from build123d import *

# Parameters (mm, degrees)
SKETCH1_W           = 51
SKETCH1_H           = 45
BOSS_EXTRUDE1_DEPTH = 5
SKETCH2_W           = 30
SKETCH2_H           = 30
BOSS_EXTRUDE2_DEPTH = 30
SKETCH3_W           = 20.5
SKETCH3_H           = 20.5
CUT_EXTRUDE1_DEPTH  = 38.5
SKETCH4_R           = 2.75
CUT_EXTRUDE2_DEPTH  = 36


with BuildPart() as part:
    # Sketch1 → Boss-Extrude1 (new body)
    with BuildSketch(Plane.XY):
        with Locations((0, -37.5)):
            Rectangle(SKETCH1_W, SKETCH1_H)
    extrude(amount=BOSS_EXTRUDE1_DEPTH)

    # Sketch2 → Boss-Extrude2 (add)
    with BuildSketch(Plane.XY.offset(5)):
        with Locations((0, -37.5)):
            Rectangle(SKETCH2_W, SKETCH2_H)
    extrude(amount=BOSS_EXTRUDE2_DEPTH)

    # Sketch3 → Cut-Extrude1 (cut, through all)
    with BuildSketch(Plane.XZ.offset(52.5)):
        with Locations((0, 20)):
            Rectangle(SKETCH3_W, SKETCH3_H)
    extrude(amount=-CUT_EXTRUDE1_DEPTH, mode=Mode.SUBTRACT)

    # Sketch4 → Cut-Extrude2 (cut, through all)
    with BuildSketch(Plane(origin=(0, 0, 0), x_dir=(-1, 0, 0), z_dir=(0, 0, -1))):
        with Locations((20, -37.5)):
            Circle(SKETCH4_R)
        with Locations((-20, -37.5)):
            Circle(SKETCH4_R)
    extrude(amount=-CUT_EXTRUDE2_DEPTH, mode=Mode.SUBTRACT)


solid = part.part
Model file for the job. Use its own axes, mm. A direction names the side the tool comes from. Give positions to 0.01 mm unless a question says otherwise; leave off trailing zeros. Loops run counter-clockwise (first coordinate to the right, second up) from the corner with the lowest first, then second, coordinate; pieces in that order, holes last. Notation, with made-up numbers: (-13, 80.5) -> (-4, 80.5) arc R7 ccw to (-4, 88.5) -> close; hole circle Ø2 at (18, 73.5). An arc over 180 degrees is marked (long way). Use a Markdown table: item, result. Add a question column.
(1) Wall check: line 1 along Z through (x, y) = (-8, -51); line 2 along X through (y, z) = (-39, 22.5); line 3 along Y through (x, z) = (20, 2). Give the ranges that are in metal, low to high.
(2) Slice it at D-D on y = -33. List the corners of the cut face in (x, z), and give its area (3 significant figures).
(3) Drop flat-ended pins along their axis: pin 1 Ø4 at (y, z) = (-47, 28.5) entering from -X; pin 2 Ø12 at (y, z) = (-42.5, 25.5) entering from +X; pin 3 Ø3 at (x, z) = (-11, 30) entering from +Y. Give the stop position or say it passes through.
(4) Mould opens along X. For faces 1 (the flat face through (0, -22, 5)), 2 (the flat face through (10.25, -38, 20)), 3 (the flat face through (25.5, -38, 2)) say: +X half, -X half, draft (parallel to the pull), parting line (faces both ways), or undercut.
(5) Slice it at B-B on x = -20. List the corners of the cut face in (y, z), and give its area (4 significant figures).
(6) Slice it at C-C on z = 22.5. List the corners of the cut face in (x, y), and give its area (3 significant figures).
(7) Tool access for faces 4 (the flat face through (15, -38, 20)), 5 (the flat face through (-15, -38, 20)), 6 (the flat face through (-10.25, -38, 20)): list every direction of +Z, -Z, +X, -X, +Y, -Y with a clear straight run to the whole face (end or side of a thin tool).
(8) Slice it at A-A on y = -37.5. List the corners of the cut face in (x, z), and give its area (3 significant figures).
Filled sheet:
| question | item | result |
|---|---|---|
| 1 | line 1 | 0 to 9.75, 30.25 to 35 |
| 1 | line 2 | -15 to -10.25, 10.25 to 15 |
| 1 | line 3 | -60 to -40.25, -34.75 to -15 |
| 2 | outline | (-25.5, 0) -> (25.5, 0) -> (25.5, 5) -> (15, 5) -> (15, 35) -> (-15, 35) -> (-15, 5) -> (-25.5, 5) -> close; hole (-10.25, 9.75) -> (10.25, 9.75) -> (10.25, 30.25) -> (-10.25, 30.25) -> close |
| 2 | area | 735 mm2 |
| 3 | pin 1 | x = -15 |
| 3 | pin 2 | x = 15 |
| 3 | pin 3 | y = -22.5 |
| 4 | face 1 | draft |
| 4 | face 2 | undercut |
| 4 | face 3 | +X half |
| 5 | outline | (-60, 0) -> (-40.25, 0) -> (-40.25, 5) -> (-60, 5) -> close; (-34.75, 0) -> (-15, 0) -> (-15, 5) -> (-34.75, 5) -> close |
| 5 | area | 197.5 mm2 |
| 6 | outline | (-15, -52.5) -> (-10.25, -52.5) -> (-10.25, -22.5) -> (-15, -22.5) -> close; (10.25, -52.5) -> (15, -52.5) -> (15, -22.5) -> (10.25, -22.5) -> close |
| 6 | area | 285 mm2 |
| 7 | face 4 | +Z, +X, +Y, -Y |
| 7 | face 5 | +Z, -X, +Y, -Y |
| 7 | face 6 | +Y, -Y |
| 8 | outline | (-25.5, 0) -> (-22.75, 0) -> (-22.75, 5) -> (-25.5, 5) -> close; (-17.25, 0) -> (17.25, 0) -> (17.25, 5) -> (15, 5) -> (15, 35) -> (-15, 35) -> (-15, 5) -> (-17.25, 5) -> close; (22.75, 0) -> (25.5, 0) -> (25.5, 5) -> (22.75, 5) -> close; hole (-10.25, 9.75) -> (10.25, 9.75) -> (10.25, 30.25) -> (-10.25, 30.25) -> close |
| 8 | area | 680 mm2 |
